Could you check a few things on this drawing? It's one solid part, dimensions in mm from its lowest x, y, z. A direction names the side the tool comes from. Give positions to 0.01 mm unless a question says otherwise; leave off trailing zeros. Order: outer loops, then holes, each group sorted by start corner. A loop starts at its lowest first (then second) coordinate and runs counter-clockwise, first axis right, second up. Notation, with made-up numbers: (52.25, 18) - (70.25, 18) arc R12 cw to (70.25, 41) - close; hole circle Ø3 at (11, 86). An arc over 180 degrees is marked (long way). One line per question, with ' | ' between items. Start each with the question number.
1. Which directions (+Z, -Z, +X, -X, +Y, -Y) give clear straight access to the entire face, cutting with the end or side of a thin tool? Please do the marked faces 1 and 2.
2. Imagine slicing it at A-A (z = 6.5). Please give me the cut outline in (x, y).
3. For P1, Ø10, axis at x = 15, z = 11, coming from the +Y side; P2, Ø1, axis at x = 15, y = 4, coming from the -Z side, each with a flat end and sliding along its axis, tell me the tip position at first contact or that it passes through.
4. Imagine slicing it at D-D (x = 44). Please give me the cut outline in (y, z).
5. Imagine slicing it at C-C (z = 10). Please give me the cut outline in (x, y).
6. I need wall thicknesses on probe 1 along X at (y, z) = (0.7, 10); probe 2 along X at (y, z) = (0.4, 6.5); probe 3 along Y at (x, z) = (13.5, 11.5). Which ranges of each line are inside material? Lowest first, please. Write a range as from..to.
7. Imagine slicing it at B-B (x = 38). Please give me the cut outline in (y, z), and give its area (3 significant figures).
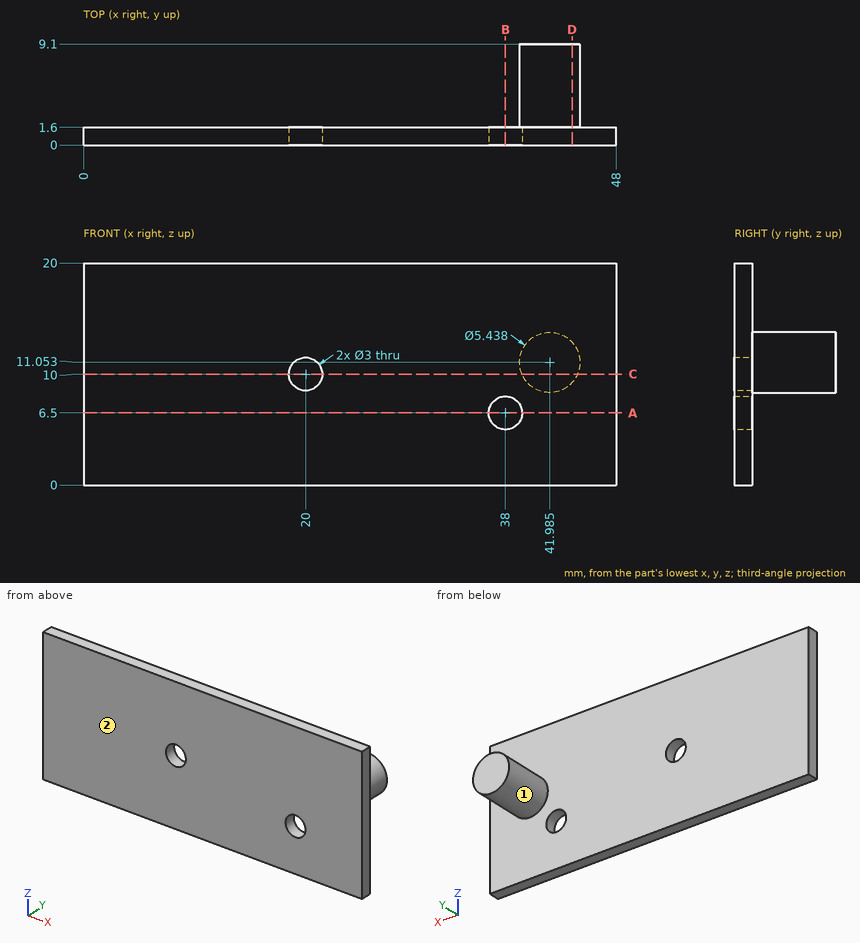
Results found:
1) face 1: +Y | face 2: +Z, -Z, +X, -X, -Y
2) outline: (0, 0) - (36.5, 0) - (36.5, 1.6) - (0, 1.6) - close; (39.5, 0) - (48, 0) - (48, 1.6) - (39.5, 1.6) - close
3) P1: stops at y = 1.6 | P2: passes through
4) outline: (0, 0) - (1.6, 0) - (1.6, 9.23) - (9.1, 9.23) - (9.1, 12.88) - (1.6, 12.88) - (1.6, 20) - (0, 20) - close
5) outline: (0, 0) - (18.5, 0) - (18.5, 1.6) - (0, 1.6) - close; (21.5, 0) - (48, 0) - (48, 1.6) - (44.49, 1.6) - (44.49, 9.1) - (39.48, 9.1) - (39.48, 1.6) - (21.5, 1.6) - close
6) probe 1: x = 0..18.5, 21.5..48 | probe 2: x = 0..36.5, 39.5..48 | probe 3: y = 0..1.6
7) outline: (0, 0) - (1.6, 0) - (1.6, 5) - (0, 5) - close; (0, 8) - (1.6, 8) - (1.6, 20) - (0, 20) - close | area: 27.2 mm2
